Print and shaded views of the part. All mm, measured from the part's lowest x, y and z. A direction names the side the tool comes from. Coordinates: 2 decimals unless noted, no trailing zeros. Order: outer loops, then holes, each group sorted by start corner. A loop starts at its lowest first (then second) coordinate and runs counter-clockwise, first axis right, second up. Notation, with made-up numbers: (-29.75, 46.25) - (-21.75, 46.25) arc R29 ccw to (-21.75, 80.25) - close; hole circle Ø10 at (11, 32). An arc over 180 degrees is marked (long way). Write each question's results on one line, items separated by ' | '.
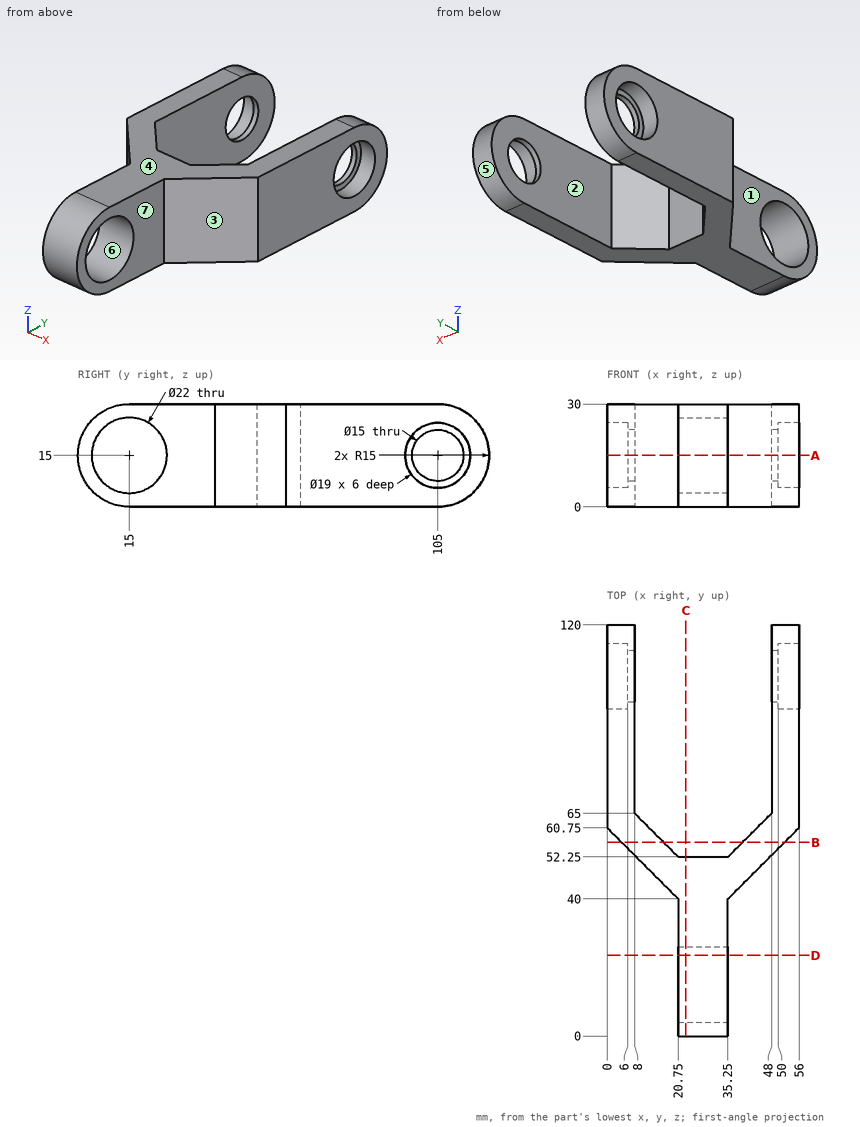
1. Drop flat-ended pins along their axis: pin 1 Ø1 at (x, z) = (37, 12) entering from +Y; pin 2 Ø11.5 at (y, z) = (105, 15) entering from -X; pin 3 Ø1 at (x, z) = (16, 11.5) entering from -Y; pin 4 Ø1 at (y, z) = (31.5, 23.5) entering from +X. Give the stop position or say it passes through.
Solved:
pin 1: stops at y = 54.5 | pin 2: passes through | pin 3: stops at y = 44.25 | pin 4: stops at x = 35.25
2. Probe line 1 (Z direction, x = 2, y = 105); line 2 (X direction, y = 71.5, z = 22.5); line 3 (X direction, y = 103, z = 6). List the from-to ranges inside material, lowest first.
Solved:
line 1: z = 0 to 5.5, 24.5 to 30 | line 2: x = 0 to 8, 48 to 56 | line 3: x = 6 to 8, 48 to 50
3. Band-saw the part on D-D on y = 23.5. Give the cut face in (x, z), then the cut area to 3 significant figures.
Solved:
outline: (20.75, 0) - (35.25, 0) - (35.25, 8.02) - (20.75, 8.02) - close; (20.75, 21.98) - (35.25, 21.98) - (35.25, 30) - (20.75, 30) - close | area: 233 mm2
4. Band-saw the part on C-C on x = 23. Give the cut face in (y, z), then the cut area to 3 significant figures.
Solved:
outline: (15, 0) - (52.25, 0) - (52.25, 30) - (15, 30) arc R15 ccw to start; hole circle Ø22 at (15, 15) | area: 1,090 mm2
5. Tool access for the marked faces 1, 2 and 3: list every direction of +Z, -Z, +X, -X, +Y, -Y with a clear straight run to the whole face (end or side of a thin tool).
Solved:
face 1: +Z, -Z, -X, -Y | face 2: +Z, -Z, +Y | face 3: +Z, -Z, +X, -Y
6. Band-saw the part on A-A on z = 15. Give the number of separate pieces and of enclosed holes in the cut face, then the cut area to 4 significant figures.
Solved:
separate pieces: 4 | enclosed holes: 0 | area: 1,475 mm2
7. Band-saw the part on B-B on y = 56.5. Give the cut face in (x, z), then the cut area to 3 significant figures.
Solved:
outline: (4.25, 0) - (16.5, 0) - (16.5, 30) - (4.25, 30) - close; (39.5, 0) - (51.75, 0) - (51.75, 30) - (39.5, 30) - close | area: 735 mm2
8. Two-plate mould, pull along Z, no slides. Class the marked faces 4, 5, 6 and 7: +Z half, -Z half, draft (parallel to the pull), parting line (faces both ways), or undercut.
Solved:
face 4: +Z half | face 5: parting line | face 6: undercut | face 7: draft
